For this review, take the finished solid that the model builds, in its own axes (mm). Face numbers are marked on the shaded views. A direction names the side the tool comes from. Coordinates: 2 decimals unless noted, no trailing zeros. Write each loop counter-clockwise with the first axis right and the second up, starting at its lowest first coordinate (ties: lowest second). Pieces come first, ordered by that corner, then holes.
1) We need section C-C on x = 60. Write out the cut boundary in (y, z).
2) For the marked faces 4, 5 and 6, list the 3-axis set-ups (+Z, -Z, +X, -X, +Y, -Y) from which the entire face can be reached by the end or side of a thin tool; tool diameter is ignored.
3) We need section B-B on z = -16. Write out the cut boundary in (x, y).
4) Insertion check: P1, Ø8, axis at x = 64, y = 15.5, coming from the -Z side; P2, Ø2, axis at x = 68.5, z = -27.5, coming from the -Y side; P3, Ø6.5, axis at x = 47.5, y = 8.5, coming from the -Z side; P4, Ø4.5, axis at x = 63.5, y = 2.5, coming from the +Z side. Each pin has a flat end and moves straight along its axis. Give the tip position at first contact, or say it passes through.
5) We need section D-D on y = 18.75. Write out the cut boundary in (x, z), then the cut area to 3 significant figures.
6) To check wall thickness, follow line 1 along Y through (x, z) = (54, -26); line 2 along Y through (x, z) = (8.5, -2); line 3 along Z through (x, y) = (47, 11.25). State the ranges of each line that lie inside material, in increasing order.
7) Mouldability with a two-part tool opening along X and no side actions: class the marked faces 1, 2 and 3 as pulls with the +X half, pulls with the -X half, needs draft (parallel to the pull), parting line crosses it, or undercut.
8) We need section A-A on y = 14. Write out the cut boundary in (x, z), then the cut area to 3 significant figures.
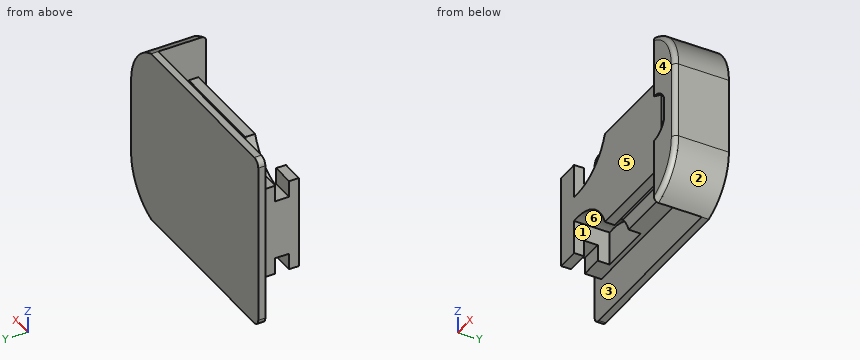
from build123d import *

# Parameters (mm, degrees)
BOSS_EXTRUDE1_DEPTH = 15.3
SKETCH4_W           = 7
SKETCH4_H           = 5.9
CUT_EXTRUDE1_DEPTH  = 78.461901488
SKETCH5_W           = 74.8
SKETCH5_H           = 19.8
BOSS_EXTRUDE2_DEPTH = 2
SKETCH6_W           = 74.8
SKETCH6_H           = 3
BOSS_EXTRUDE3_DEPTH = 37.2
SKETCH7_W           = 37.2
SKETCH7_H           = 3
BOSS_EXTRUDE4_DEPTH = 5
FILLET1_R           = 3
BOSS_EXTRUDE5_DEPTH = 23.3
FILLET2_R           = 2
SKETCH10_W          = 74.8
SKETCH10_H          = 19.8
CUT_EXTRUDE2_DEPTH  = 0.2
CUT_EXTRUDE3_DEPTH  = 5
CUT_EXTRUDE3_DRAFT  = 30
BOSS_EXTRUDE6_DEPTH = 15


with BuildPart() as part:
    # Sketch1 → Boss-Extrude1 (new body)
    with BuildSketch(Plane(origin=(0, 0, 0), x_dir=(1, 0, 0), z_dir=(0, 1, 0))):
        with BuildLine():
            Line((1.005677457, 13.08496015), (1.005677457, -6.71503985))
            Line((1.005677457, -6.71503985), (10.705677457, -6.71503985))
            Line((10.705677457, -6.71503985), (10.705677457, 7.68496015))
            ThreePointArc((10.705677457, 7.68496015), (24.690281417, 4.453424809), (33.705677457, -6.71503985))
            Line((33.705677457, -6.71503985), (75.805677457, -6.71503985))
            Line((75.805677457, -6.71503985), (75.805677457, 13.08496015))
            Line((75.805677457, 13.08496015), (1.005677457, 13.08496015))
        make_face()
    extrude(amount=BOSS_EXTRUDE1_DEPTH)

    # Sketch4 → Cut-Extrude1 (cut, through all)
    with BuildSketch(Plane(origin=(75.805677457, 0, 0), x_dir=(0, 0, -1), z_dir=(1, 0, 0))):
        with Locations((-3.21503985, 7.3)):
            Rectangle(SKETCH4_W, SKETCH4_H)
    extrude(amount=-CUT_EXTRUDE1_DEPTH, mode=Mode.SUBTRACT)

    # Sketch5 → Boss-Extrude2 (add)
    with BuildSketch(Plane(origin=(0, 15.3, 0), x_dir=(1, 0, 0), z_dir=(0, 1, 0))):
        with Locations((38.405677457, 3.18496015)):
            Rectangle(SKETCH5_W, SKETCH5_H)
    extrude(amount=BOSS_EXTRUDE2_DEPTH)

    # Sketch6 → Boss-Extrude3 (add)
    with BuildSketch(Plane(origin=(0, 0, -13.08496015), x_dir=(-1, 0, 0), z_dir=(0, 0, -1))):
        with Locations((-38.405677457, 18.8)):
            Rectangle(SKETCH6_W, SKETCH6_H)
    extrude(amount=-BOSS_EXTRUDE3_DEPTH)

    # Sketch7 → Boss-Extrude4 (add)
    with BuildSketch(Plane.ZY.offset(-1.005677457)):
        with Locations((5.51503985, 18.8)):
            Rectangle(SKETCH7_W, SKETCH7_H)
    extrude(amount=BOSS_EXTRUDE4_DEPTH)

    # Fillet1
    fillet1_edges = [part.edges().sort_by_distance(p)[0] for p in [
        (-3.994322543, 18.8, 24.11503985),
    ]]
    fillet(fillet1_edges, radius=FILLET1_R)

    # Sketch8 → Boss-Extrude5 (add)
    with BuildSketch(Plane(origin=(0, 20.3, 0), x_dir=(1, 0, 0), z_dir=(0, 1, 0))):
        with BuildLine():
            Line((75.805677457, 13.08496015), (90.805677457, 13.08496015))
            Line((90.805677457, 13.08496015), (90.805677457, -3.072659154))
            ThreePointArc((90.805677457, -3.072659154), (86.671822493, -15.993396221), (75.805677457, -24.11503985))
            Line((75.805677457, -24.11503985), (75.805677457, 13.08496015))
        make_face()
    extrude(amount=-BOSS_EXTRUDE5_DEPTH)

    # Fillet2
    fillet2_edges = [part.edges().sort_by_distance(p)[0] for p in [
        (90.805677457, -3, -5.006150498),
        (86.671822493, -3, 15.993396221),
    ]]
    fillet(fillet2_edges, radius=FILLET2_R)

    # Sketch10 → Cut-Extrude2 (cut)
    with BuildSketch(Plane(origin=(0, 0, 0), x_dir=(-1, 0, 0), z_dir=(0, -1, 0))):
        with Locations((-38.405677457, 3.18496015)):
            Rectangle(SKETCH10_W, SKETCH10_H)
    extrude(amount=-CUT_EXTRUDE2_DEPTH, mode=Mode.SUBTRACT)


with BuildPart() as cut_extrude3_tool:
    # Sketch11 → Cut-Extrude3 (with draft: the straight prism first)
    with BuildSketch(Plane(origin=(0, -3, 0), x_dir=(-1, 0, 0), z_dir=(0, -1, 0))):
        with BuildLine():
            Line((-75.805677457, 13.08496015), (-83.305677457, 13.08496015))
            Line((-83.305677457, 13.08496015), (-83.305677457, 8.08496015))
            ThreePointArc((-83.305677457, 8.08496015), (-80.312616551, 4.449551508), (-75.805677457, 3.08496015))
            Line((-75.805677457, 3.08496015), (-75.805677457, 13.08496015))
        make_face()
    extrude(amount=-CUT_EXTRUDE3_DEPTH)
    # Cut-Extrude3: the draft: its side faces are tilted about the plane it starts from
    cut_extrude3_sides = [cut_extrude3_tool.faces().sort_by_distance(p)[0] for p in [
        (75.805677457, -0.5, -8.08496015),
        (79.555677457, -0.5, -13.08496015),
        (83.305677457, -0.5, -10.58496015),
        (80.312616551, -0.5, -4.449551508),
    ]]
    draft(cut_extrude3_sides, Plane(origin=(0, -3, 0), x_dir=(-1, 0, 0), z_dir=(0, -1, 0)), CUT_EXTRUDE3_DRAFT)


with BuildPart() as part_1:
    add(part.part)

    # Cut-Extrude3: cut by cut_extrude3_tool
    add(cut_extrude3_tool.part, mode=Mode.SUBTRACT)

    # Sketch14 → Boss-Extrude6 (add)
    with BuildSketch(Plane(origin=(0, 0, -13.08496015), x_dir=(-1, 0, 0), z_dir=(0, 0, -1))):
        Polygon((-72.918926111, 2), (-73.958156595, 0.2), (-75.805677457, 0.2), (-75.805677457, 2), align=None)
    extrude(amount=-BOSS_EXTRUDE6_DEPTH)

    # Mirror1: part across plane


with BuildPart() as part_2:
    add(part_1.part)
    add(part_1.part.mirror(Plane(origin=(0, 15.3, -13.08496015), x_dir=(1, 0, 0), z_dir=(0, 0, -1))))


solid = part_2.part
Result:
1. outline: (0.2, -32.88) - (4.35, -32.88) - (4.35, -25.88) - (10.25, -25.88) - (10.25, -32.88) - (17.3, -32.88) - (17.3, -50.28) - (20.3, -50.28) - (20.3, 24.12) - (17.3, 24.12) - (17.3, 6.72) - (10.25, 6.72) - (10.25, -0.28) - (4.35, -0.28) - (4.35, 6.72) - (0.2, 6.72) - close
2. face 4: +Z, -Z, +X, -X, -Y
2. face 5: +Z, -Z, -X, -Y
2. face 6: -Z, -Y
3. outline: (-3.99, 17.3) - (1.01, 17.3) - (1.01, 0.2) - (75.81, 0.2) - (75.81, 2) - (86.19, 2) - (83.31, -3) - (88.81, -3) arc R2 ccw to (90.81, -1) - (90.81, 20.3) - (-3.99, 20.3) - close
4. P1: stops at z = -50.28
4. P2: stops at y = 0.2
4. P3: stops at z = -32.88
4. P4: stops at z = 6.72
5. outline: (-3.99, -47.28) arc R3 ccw to (-0.99, -50.28) - (75.81, -50.28) arc R22.26 ccw to (90.81, -29.24) - (90.81, 3.07) arc R22.26 ccw to (75.81, 24.12) - (-0.99, 24.12) arc R3 ccw to (-3.99, 21.12) - close
5. area: 6,880 mm2
6. line 1: y = 0.2 to 4.35, 10.25 to 20.3
6. line 2: y = 0.2 to 20.3
6. line 3: z = -32.88 to 6.72
7. face 1: undercut
7. face 2: pulls with the +X half
7. face 3: needs draft
8. outline: (1.01, -32.88) - (10.71, -32.88) - (10.71, -18.48) arc R22 cw to (33.71, -32.88) - (75.81, -32.88) - (75.81, -50.28) arc R22.26 ccw to (90.81, -29.24) - (90.81, 3.07) arc R22.26 ccw to (75.81, 24.12) - (75.81, 6.72) - (33.71, 6.72) arc R22 cw to (10.71, -7.68) - (10.71, 6.72) - (1.01, 6.72) - close
8. area: 3,400 mm2
